Geometry check sheet. Reference: the model listing, model coordinates, mm. A direction names the side the tool comes from. Give positions to 0.01 mm unless a question says otherwise; leave off trailing zeros. Write each loop counter-clockwise with the first axis right and the second up, starting at its lowest first coordinate (ties: lowest second). Pieces come first, ordered by that corner, then holes.
(1) Mould release check, pull along Y, two halves, no side actions. Record for faces 1 (the flat face through (-24.406, 1, 1)), 2 (the cylindrical face through (-48.68, -8.65, 1.48)), 3 (the flat face through (-13, 12, 3)): +Y half, -Y half, draft (parallel to the pull), parting line (faces both ways), or undercut.
(2) Cross-section at C-C (y = 0.75). Record the boundary of the cut face in (x, z), and give its area (3 significant figures).
(3) Tool access check on faces 4 (the flat face through (20, -7.764, 1)), 5 (the flat face through (-2, -9.25, 1)). Record the directions out of +Z, -Z, +X, -X, +Y, -Y that give a thin tool (end or side, any length) a straight path to the whole face; none if there is none.
(4) Cross-section at A-A (x = 33.5). Record the boundary of the cut face in (y, z).
(5) Depth check by flat-ended pin: P1, Ø5, axis at x = -36.5, y = 0.75, coming from the +Z side. Enter the tip coordinate at first touch or a pass-through.
(6) Thickness scan on line 1 along Y through (x, z) = (-36.5, 0.85); line 2 along Y through (x, z) = (20, 0.3); line 3 along X through (y, z) = (7.25, 2.2). Record the ranges inside material, lowest first.
```python
from build123d import *

# Parameters (mm, degrees)
SKETCH1_R           = 3
BOSS_EXTRUDE1_DEPTH = 3


with BuildPart() as part:
    # Sketch1 → Boss-Extrude1 (new body)
    with BuildSketch(Plane.XY):
        with BuildLine():
            ThreePointArc((46, 17.75), (45.414213562, 19.164213562), (44, 19.75))
            Line((44, 19.75), (-47.25, 19.75))
            ThreePointArc((-47.25, 19.75), (-48.664213562, 19.164213562), (-49.25, 17.75))
            Line((-49.25, 17.75), (-49.25, -7.25))
            ThreePointArc((-49.25, -7.25), (-48.664213562, -8.664213562), (-47.25, -9.25))
            Line((-47.25, -9.25), (44, -9.25))
            ThreePointArc((44, -9.25), (45.219142744, -8.835462384), (45.932904961, -7.763690971))
            Line((45.932904961, -7.763690971), (45.906437474, -7.763690971))
            Line((45.906437474, -7.763690971), (28.406437474, -7.763690971))
            Line((28.406437474, -7.763690971), (28.092497309, -7.763690971))
            Line((28.092497309, -7.763690971), (10.906437474, -7.763690971))
            Line((10.906437474, -7.763690971), (10.592497309, -7.763690971))
            Line((10.592497309, -7.763690971), (-6.907502691, -7.763690971))
            Line((-6.907502691, -7.763690971), (-6.907502691, -7.736309029))
            Line((-6.907502691, -7.736309029), (-24.406437474, -7.736309029))
            Line((-24.406437474, -7.736309029), (-24.406437474, 9.263690971))
            Line((-24.406437474, 9.263690971), (-6.592497309, 9.263690971))
            Line((-6.592497309, 9.263690971), (-6.592497309, 9.236309029))
            Line((-6.592497309, 9.236309029), (10.592497309, 9.236309029))
            Line((10.592497309, 9.236309029), (10.906437474, 9.236309029))
            Line((10.906437474, 9.236309029), (28.092497309, 9.236309029))
            Line((28.092497309, 9.236309029), (28.406437474, 9.236309029))
            Line((28.406437474, 9.236309029), (45.906437474, 9.236309029))
            Line((45.906437474, 9.236309029), (46, 9.236309029))
            Line((46, 9.236309029), (46, 17.75))
        make_face()
        with Locations((-36.5, 0.75)):
            Circle(SKETCH1_R, mode=Mode.SUBTRACT)
    extrude(amount=BOSS_EXTRUDE1_DEPTH)


solid = part.part
```
Reply:
1. face 1: undercut
1. face 2: -Y half
1. face 3: draft
2. outline: (-49.25, 0) - (-39.5, 0) - (-39.5, 3) - (-49.25, 3) - close; (-33.5, 0) - (-24.41, 0) - (-24.41, 3) - (-33.5, 3) - close
2. area: 56.5 mm2
3. face 4: +Z, -Z, +X
3. face 5: +Z, -Z, +X, -X, -Y
4. outline: (-9.25, 0) - (-7.76, 0) - (-7.76, 3) - (-9.25, 3) - close; (9.24, 0) - (19.75, 0) - (19.75, 3) - (9.24, 3) - close
5. P1: passes through
6. line 1: y = -9.25 to -2.25, 3.75 to 19.75
6. line 2: y = -9.25 to -7.76, 9.24 to 19.75
6. line 3: x = -49.25 to -24.41
